For this review, take the finished solid that the model builds, in its own axes (mm). A direction names the side the tool comes from. Coordinates: 2 decimals unless noted, no trailing zeros. Loops run counter-clockwise (first coordinate to the right, second up) from the corner with the lowest first, then second, coordinate; pieces in that order, holes last.
```python
from build123d import *

# Parameters (mm, degrees)
SKETCH1_W           = 197.2
SKETCH1_H           = 25.6
SKETCH1_R           = 6.55
BOSS_EXTRUDE1_DEPTH = 1.5
SKETCH3_W           = 125
SKETCH3_H           = 25.6
SKETCH3_W_2         = 4
BOSS_EXTRUDE3_DEPTH = 2.5


with BuildPart() as part:
    # Sketch1 → Boss-Extrude1 (new body)
    with BuildSketch(Plane(origin=(0, 0, 0), x_dir=(1, 0, 0), z_dir=(0, 1, 0))):
        Rectangle(SKETCH1_W, SKETCH1_H)
        with Locations(Location((-84.25, 0, 0), (0, 0, 270))):
            Circle(SKETCH1_R, mode=Mode.SUBTRACT)
        with Locations(Location((84.25, 0, 0), (0, 0, 270))):
            Circle(SKETCH1_R, mode=Mode.SUBTRACT)
    extrude(amount=BOSS_EXTRUDE1_DEPTH)

    # Sketch3 → Boss-Extrude3 (add)
    with BuildSketch(Plane(origin=(0, 1.5, 0), x_dir=(1, 0, 0), z_dir=(0, 1, 0))):
        Rectangle(SKETCH3_W, SKETCH3_H)
        with Locations((-96.6, 0)):
            Rectangle(SKETCH3_W_2, SKETCH3_H)
        with Locations((96.6, 0)):
            Rectangle(SKETCH3_W_2, SKETCH3_H)
    extrude(amount=BOSS_EXTRUDE3_DEPTH)


solid = part.part
```
Q1. Consider section C-C (z = -9.25). State the section outline as (x, y) points.
Q2. Consider section A-A (x = 84.25). State the section outline as (y, z) points.
Q3. For pin 1 Ø13 at (x, z) = (86.5, 5) entering from +Y; pin 2 Ø3 at (x, z) = (77.5, 6) entering from -Y, all flat-tipped, find the tip position at first contact; note any pin that passes through.
Q4. Wall thickness on probe 1 along X at (y, z) = (2.8, 6.25); probe 2 along X at (y, z) = (0.5, 0); probe 3 along Y at (x, z) = (-69.5, 11.5): over which ranges is each line inside the solid? List them lowest first.
Q5. Consider section B-B (z = 0). State the section outline as (x, y) points.
Q6. The part is to be moulded in two halves that separate along Z. For faces 1 (the face through (75, 1.5, 0)), 2 (the face through (-1, 2, -12.8)), 3 (the face through (-90.644, 0.74, -1.42)), 4 (the face through (-1, 2, 12.8)), say which applies: +Z half, -Z half, draft (parallel to the pull), parting line (faces both ways), or undercut.
Q7. Machinability: for faces 5 (the face through (-75, 1.5, 0)), 6 (the face through (-1, 4, 0)), which of the approach directions +Z, -Z, +X, -X, +Y, -Y give a long, thin tool a straight path to every point of the face, cutting with its end or side? Answer none if there is none.
Model answer:
1. outline: (-98.6, 0) - (98.6, 0) - (98.6, 4) - (94.6, 4) - (94.6, 1.5) - (62.5, 1.5) - (62.5, 4) - (-62.5, 4) - (-62.5, 1.5) - (-94.6, 1.5) - (-94.6, 4) - (-98.6, 4) - close
2. outline: (0, -12.8) - (1.5, -12.8) - (1.5, -6.55) - (0, -6.55) - close; (0, 6.55) - (1.5, 6.55) - (1.5, 12.8) - (0, 12.8) - close
3. pin 1: stops at y = 1.5
3. pin 2: stops at y = 0
4. probe 1: x = -98.6 to -94.6, -62.5 to 62.5, 94.6 to 98.6
4. probe 2: x = -98.6 to -90.8, -77.7 to 77.7, 90.8 to 98.6
4. probe 3: y = 0 to 1.5
5. outline: (-98.6, 0) - (-90.8, 0) - (-90.8, 1.5) - (-94.6, 1.5) - (-94.6, 4) - (-98.6, 4) - close; (-77.7, 0) - (77.7, 0) - (77.7, 1.5) - (62.5, 1.5) - (62.5, 4) - (-62.5, 4) - (-62.5, 1.5) - (-77.7, 1.5) - close; (90.8, 0) - (98.6, 0) - (98.6, 4) - (94.6, 4) - (94.6, 1.5) - (90.8, 1.5) - close
6. face 1: draft
6. face 2: -Z half
6. face 3: undercut
6. face 4: +Z half
7. face 5: +Z, -Z, +Y
7. face 6: +Z, -Z, +X, -X, +Y
